Design review of the part built by this model. Coordinates are the model's own, in mm. A direction names the side the tool comes from. Coordinates: 2 decimals unless noted, no trailing zeros. Write each loop counter-clockwise with the first axis right and the second up, starting at its lowest first coordinate (ties: lowest second). Pieces come first, ordered by that corner, then holes.
Q1. The part is to be moulded in two halves that separate along Y. For faces 1 (the face through (35, 0, 10)), 2 (the face through (77, -90, 0)), 3 (the face through (80, -77.274, 10)), say which applies: +Y half, -Y half, draft (parallel to the pull), parting line (faces both ways), or undercut.
Q2. Add section B-B, the plane z = 8. Give the boundary of the cut face in (x, y), plus the area to 3 significant figures.
Q3. Add section C-C, the plane x = 279. Give the boundary of the cut face in (y, z), plus the area to 3 significant figures.
Q4. Add section A-A, the plane y = -165. Give the boundary of the cut face in (x, z).
Q5. Add section D-D, the plane y = -136. Give the boundary of the cut face in (x, z), plus the area to 3 significant figures.
Q6. Machinability: for faces 4 (the face through (79, -154.548, 10)), 5 (the face through (57.5, -55, 10)), 6 (the face through (207.62, -12.76, 10.14)), 7 (the face through (70, -16, 10)), 8 (the face through (77, -90, 20)), which of the approach directions +Z, -Z, +X, -X, +Y, -Y give a long, thin tool a straight path to every point of the face, cutting with its end or side? Answer none if there is none.
Q7. To check wall thickness, follow probe 1 along Y at (x, z) = (105.5, 2); probe 2 along X at (y, z) = (-104, 5.5); probe 3 along X at (y, z) = (-58.5, 11.5). State the ranges of each line that lie inside material, in increasing order.
Q8. Clearance check with flat-ended pins moving along their axes: pin 1 Ø3 at (y, z) = (-36.5, 9) entering from +X; pin 2 Ø1.5 at (x, z) = (237, 16.5) entering from +Y; pin 3 Ø2 at (y, z) = (-50.5, 9) entering from +X. State where each tip first meets the part, or that it passes through.
Autodesk Inventor part; units mm, degrees
ref_plane "YZ Plane" through (0, 0, 0) normal (1, 0, 0) x (0, 1, 0)
ref_plane "XZ Plane" through (0, 0, 0) normal (0, 1, 0) x (-1, 0, 0)
ref_plane "XY Plane" through (0, 0, 0) normal (0, 0, 1) x (1, 0, 0)
sketch "Sketch1" plane through (0, 0, 0) normal (0, 0, 1) x (1, 0, 0)
  line L0 (0, 0) -> (160, 0)
  line L1 (160, 0) -> (118.589, -154.5481)
  line L2 (0, 0) -> (41.411, -154.5481)
  line L3 (41.411, -154.5481) -> (118.589, -154.5481)
  dimension "d0" = 160
  dimension "d1" = 160
  dimension "d2" = 160
  dimension "d3" = 75
  dimension "d4" = 75
extrude "Extrusion1" add sketch "Sketch1" along normal blind 20
sketch "Sketch3" plane through (0, 0, 20) normal (0, 0, 1) x (1, 0, 0)
  line L0 (57.5, -32.2741) -> (102.5, -32.2741)
  line L1 (102.5, -32.2741) -> (102.5, -77.2741)
  line L2 (102.5, -77.2741) -> (57.5, -77.2741)
  line L3 (57.5, -77.2741) -> (57.5, -32.2741)
  line L4 (0, 0) -> (41.411, -154.5481)
  line L5 (160, 0) -> (0, 0)
  line L6 (70, 0) -> (90, 0)
  line L7 (90, 0) -> (90, -32.2741)
  line L8 (90, -32.2741) -> (70, -32.2741)
  line L9 (70, -32.2741) -> (70, 0)
  point P0 (20.7055, -77.2741)
  point P1 (80, 0)
  point P2 (80, -32.2741)
  point P3 (80, -32.2741)
  point P4 (80, 0)
  dimension "d10" = 45
  dimension "d11" = 45
  dimension "d14" = 20
extrude "Extrusion3" cut sketch "Sketch3" against normal blind 40
sketch "Sketch4" plane through (0, 0, 20) normal (0, 0, 1) x (1, 0, 0)
  line L0 (70, -32.2741) -> (70, 0)
  line L1 (70, 0) -> (0, 0)
  line L2 (0, 0) -> (41.411, -154.5481)
  line L3 (41.411, -154.5481) -> (118.589, -154.5481)
  line L4 (118.589, -154.5481) -> (160, 0)
  line L5 (160, 0) -> (90, 0)
  line L6 (90, 0) -> (90, -32.2741)
  line L7 (90, -32.2741) -> (102.5, -32.2741)
  line L8 (102.5, -32.2741) -> (102.5, -77.2741) construction
  line L9 (102.5, -77.2741) -> (57.5, -77.2741)
  line L10 (57.5, -77.2741) -> (57.5, -32.2741)
  line L11 (57.5, -32.2741) -> (70, -32.2741)
  line L12 (57.5, -77.2741) -> (102.5, -77.2741) construction
  line L13 (102.5, -77.2741) -> (102.5, -32.2741)
  line L14 (102.5, -32.2741) -> (57.5, -32.2741) construction
  line L15 (57.5, -32.2741) -> (57.5, -77.2741) construction
  line L16 (57.5, -77.2741) -> (102.5, -32.2741) construction
  line L17 (102.5, -77.2741) -> (57.5, -32.2741) construction
  circle A0 centre (80, -19.7741) radius 2.5
  circle A1 centre (49.6891, -37.2741) radius 2.5
  circle A2 centre (49.6891, -72.2741) radius 2.5
  circle A3 centre (80, -89.7741) radius 2.5
  circle A4 centre (110.3109, -72.2741) radius 2.5
  circle A5 centre (110.3109, -37.2741) radius 2.5
  point P0 (80, -54.7741)
  point P1 (80, -54.7741)
  dimension "d15" = 45
  dimension "d16" = 45
  dimension "d17" = 5
  dimension "d18" = 35
  dimension "d21" = 360
extrude "Extrusion4" cut sketch "Sketch4" against normal through all contours A1 | A2 | A3 | A4 | A5
sketch "Sketch5" plane through (0, 0, 20) normal (0, 0, 1) x (1, 0, 0)
  line L0 (160, 0) -> (90, 0)
  line L1 (160, 0) -> (256.5926, -25.8819)
  line L2 (118.589, -154.5481) -> (41.411, -154.5481)
  line L3 (118.589, -154.5481) -> (215.1815, -180.43)
  circle A0 centre (235.8871, -103.156) radius 80 construction
  arc A1 (215.1815, -180.43) -> (256.5926, -25.8819) centre (235.8871, -103.156) ccw
  line L4 (160, 0) -> (118.589, -154.5481)
  line L5 (0, 0) -> (41.411, -154.5481)
  line L6 (0, 0) -> (-96.5926, -25.8819)
  line L7 (41.411, -154.5481) -> (118.589, -154.5481)
  line L8 (41.411, -154.5481) -> (-55.1815, -180.43)
  circle A2 centre (-75.8871, -103.156) radius 80 construction
  arc A3 (-96.5926, -25.8819) -> (-55.1815, -180.43) centre (-75.8871, -103.156) ccw
  dimension "d25" = 100
  dimension "d26" = 100
  dimension "d27" = 160
  dimension "d30" = 100
  dimension "d31" = 100
  dimension "d32" = 160
extrude "Extrusion5" add sketch "Sketch5" against normal blind 20
properties part number "HA002" material "ABS Plastic"
Here are the results:
1. face 1: +Y half
1. face 2: draft
1. face 3: undercut
2. outline: (-96.59, -25.88) arc R80 ccw to (-55.18, -180.43) - (41.41, -154.55) - (118.59, -154.55) - (215.18, -180.43) arc R80 ccw to (256.59, -25.88) - (160, 0) - (90, 0) - (90, -32.27) - (102.5, -32.27) - (102.5, -77.27) - (57.5, -77.27) - (57.5, -32.27) - (70, -32.27) - (70, 0) - (0, 0) - close; hole circle Ø5 at (49.69, -72.27); hole circle Ø5 at (49.69, -37.27); hole circle Ø5 at (80, -89.77); hole circle Ø5 at (110.31, -72.27); hole circle Ø5 at (110.31, -37.27)
2. area: 67,700 mm2
3. outline: (-170.54, 0) - (-35.77, 0) - (-35.77, 20) - (-170.54, 20) - close
3. area: 2,700 mm2
4. outline: (-126.63, 0) - (2.4, 0) - (2.4, 20) - (-126.63, 20) - close; (157.6, 0) - (286.63, 0) - (286.63, 20) - (157.6, 20) - close
5. outline: (-148.83, 0) - (308.83, 0) - (308.83, 20) - (-148.83, 20) - close
5. area: 9,150 mm2
6. face 4: +Z, -Z, -Y
6. face 5: +Z, -Z
6. face 6: +Z, -Z, +X, +Y
6. face 7: +Z, -Z, +Y
6. face 8: +Z, +X, -X, +Y, -Y
7. probe 1: y = -154.55 to 0
7. probe 2: x = -155.88 to 315.88
7. probe 3: x = -142.26 to 57.5, 102.5 to 302.26
8. pin 1: stops at x = 282.31
8. pin 2: stops at y = -20.43
8. pin 3: stops at x = 296.97
